```python
from build123d import *

# Parameters (mm, degrees)
SKETCH_W     = 228
SKETCH_H     = 130
SKETCH_R     = 1.75
PAD_DEPTH    = 3
SKETCH001_W  = 5
SKETCH001_H  = 120
PAD001_DEPTH = 13
SKETCH002_R  = 1.15
POCKET_DEPTH = 112.5


with BuildPart() as part:
    # Sketch → Pad (new body)
    with BuildSketch(Plane.XY):
        with Locations((4, 0)):
            Rectangle(SKETCH_W, SKETCH_H)
        with Locations((-90, 62)):
            Circle(SKETCH_R, mode=Mode.SUBTRACT)
        with Locations((0, 62)):
            Circle(SKETCH_R, mode=Mode.SUBTRACT)
        with Locations((90, 62)):
            Circle(SKETCH_R, mode=Mode.SUBTRACT)
        with Locations((-90, -62)):
            Circle(SKETCH_R, mode=Mode.SUBTRACT)
        with Locations((0, -62)):
            Circle(SKETCH_R, mode=Mode.SUBTRACT)
        with Locations((90, -62)):
            Circle(SKETCH_R, mode=Mode.SUBTRACT)
        with BuildLine():
            ThreePointArc((-90, 43.5), (-91.75, 41.75), (-90, 40))
            Line((-90, 40), (-10, 40))
            ThreePointArc((-10, 40), (-8.25, 41.75), (-10, 43.5))
            Line((-90, 43.5), (-10, 43.5))
        make_face(mode=Mode.SUBTRACT)
        with BuildLine():
            ThreePointArc((-90, 33.5), (-91.75, 31.75), (-90, 30))
            Line((-90, 30), (-10, 30))
            ThreePointArc((-10, 30), (-8.25, 31.75), (-10, 33.5))
            Line((-90, 33.5), (-10, 33.5))
        make_face(mode=Mode.SUBTRACT)
        with BuildLine():
            ThreePointArc((-90, 23.5), (-91.75, 21.75), (-90, 20))
            Line((-90, 20), (-10, 20))
            ThreePointArc((-10, 20), (-8.25, 21.75), (-10, 23.5))
            Line((-90, 23.5), (-10, 23.5))
        make_face(mode=Mode.SUBTRACT)
        with BuildLine():
            ThreePointArc((-90, 13.5), (-91.75, 11.75), (-90, 10))
            Line((-90, 10), (-10, 10))
            ThreePointArc((-10, 10), (-8.25, 11.75), (-10, 13.5))
            Line((-90, 13.5), (-10, 13.5))
        make_face(mode=Mode.SUBTRACT)
        with BuildLine():
            ThreePointArc((-90, 3.5), (-91.75, 1.75), (-90, 0))
            Line((-90, 0), (-10, 0))
            ThreePointArc((-10, 0), (-8.25, 1.75), (-10, 3.5))
            Line((-90, 3.5), (-10, 3.5))
        make_face(mode=Mode.SUBTRACT)
    extrude(amount=PAD_DEPTH)

    # Sketch001 → Pad001 (join)
    with BuildSketch(Plane.XY):
        with Locations((104.5, 5)):
            Rectangle(SKETCH001_W, SKETCH001_H)
        with Locations((-104.5, 5)):
            Rectangle(SKETCH001_W, SKETCH001_H)
    extrude(amount=PAD001_DEPTH)

    # Sketch002 → Pocket (cut, symmetric)
    with BuildSketch(Plane.YZ):
        with Locations((-51, 7)):
            Circle(SKETCH002_R)
        with Locations((61, 7)):
            Circle(SKETCH002_R)
    extrude(amount=POCKET_DEPTH, both=True, mode=Mode.SUBTRACT)


solid = part.part
```
Read the model definition and answer for the solid it produces. Units are mm, in the model's axes. A direction names the side the tool comes from. Coordinates: 2 decimals unless noted, no trailing zeros. Write each loop counter-clockwise with the first axis right and the second up, starting at its lowest first coordinate (ties: lowest second). Pieces come first, ordered by that corner, then holes. Notation, with made-up numbers: (24.5, -1.75) -> (52.5, -1.75) arc R5 ccw to (52.5, 3.25) -> close; hole circle Ø1 at (-24.75, 16.25). An arc over 180 degrees is marked (long way). Write item = value, one per line.
(1) Which of the six approach directions +Z, -Z, +X, -X, +Y, -Y give full straight-line access (tool end or side, diameter ignored) to faces 4 (the face through (107, 4, 8)), 5 (the face through (102, 4, 8)), 6 (the face through (104, -55, 8))?
From the geometry:
face_4 = +Z, +X, +Y, -Y
face_5 = +Z, +Y, -Y
face_6 = +Z, +X, -X, -Y
(2) Section A-A on x = -26 is taken. Write down the section's boundary in (y, z), plus the area to 4 significant figures.
From the geometry:
outline = (-65, 0) -> (0, 0) -> (0, 3) -> (-65, 3) -> close; (3.5, 0) -> (10, 0) -> (10, 3) -> (3.5, 3) -> close; (13.5, 0) -> (20, 0) -> (20, 3) -> (13.5, 3) -> close; (23.5, 0) -> (30, 0) -> (30, 3) -> (23.5, 3) -> close; (33.5, 0) -> (40, 0) -> (40, 3) -> (33.5, 3) -> close; (43.5, 0) -> (65, 0) -> (65, 3) -> (43.5, 3) -> close
area = 337.5 mm2
(3) Section D-D on x = 73 is taken. Write down the section's boundary in (y, z).
From the geometry:
outline = (-65, 0) -> (65, 0) -> (65, 3) -> (-65, 3) -> close
(4) Straight lines are drawn through the part: L1, parallel to Y at x = -49, z = 2.5; L2, parallel to X at y = 47, z = 9; L3, parallel to Y at x = 0, z = 1.3. For each, find the intervals that lie inside material, in ascending order. Write a range as from..to.
From the geometry:
L1 = -65..0, 3.5..10, 13.5..20, 23.5..30, 33.5..40, 43.5..65
L2 = -107..-102, 102..107
L3 = -65..-63.75, -60.25..60.25, 63.75..65
(5) Section B-B on z = 10.5 is taken. Write down the section's boundary in (x, y).
From the geometry:
outline = (-107, -55) -> (-102, -55) -> (-102, 65) -> (-107, 65) -> close; (102, -55) -> (107, -55) -> (107, 65) -> (102, 65) -> close
(6) Given pin 1 Ø3.5 at (y, z) = (-51, 7) entering from +X; pin 2 Ø5.5 at (x, y) = (90, 62) entering from +Z; pin 3 Ø4 at (y, z) = (47, 7) entering from -X, each flat-ended and moving along its own axis, determine where each tip first touches the part or whether it passes through.
From the geometry:
pin_1 = 107
pin_2 = 3
pin_3 = -107
(7) Section C-C on y = 48 is taken. Write down the section's boundary in (x, z).
From the geometry:
outline = (-110, 0) -> (118, 0) -> (118, 3) -> (107, 3) -> (107, 13) -> (102, 13) -> (102, 3) -> (-102, 3) -> (-102, 13) -> (-107, 13) -> (-107, 3) -> (-110, 3) -> close
(8) For a pull along X with two mould halves and no side action, classify faces 1 (the face through (-102, 4, 8)), 2 (the face through (-107, 4, 8)), 3 (the face through (-105, -55, 8)) as +X half, -X half, draft (parallel to the pull), parting line (faces both ways), or undercut.
From the geometry:
face_1 = undercut
face_2 = -X half
face_3 = draft
